The figure shows three views and two pictorial views of one solid part (mm, origin at its lowest corner). Answer the questions. Coordinates: 2 decimals unless noted, no trailing zeros. Order: outer loops, then holes, each group sorted by start corner. A loop starts at its lowest first (then second) coordinate and runs counter-clockwise, first axis right, second up.
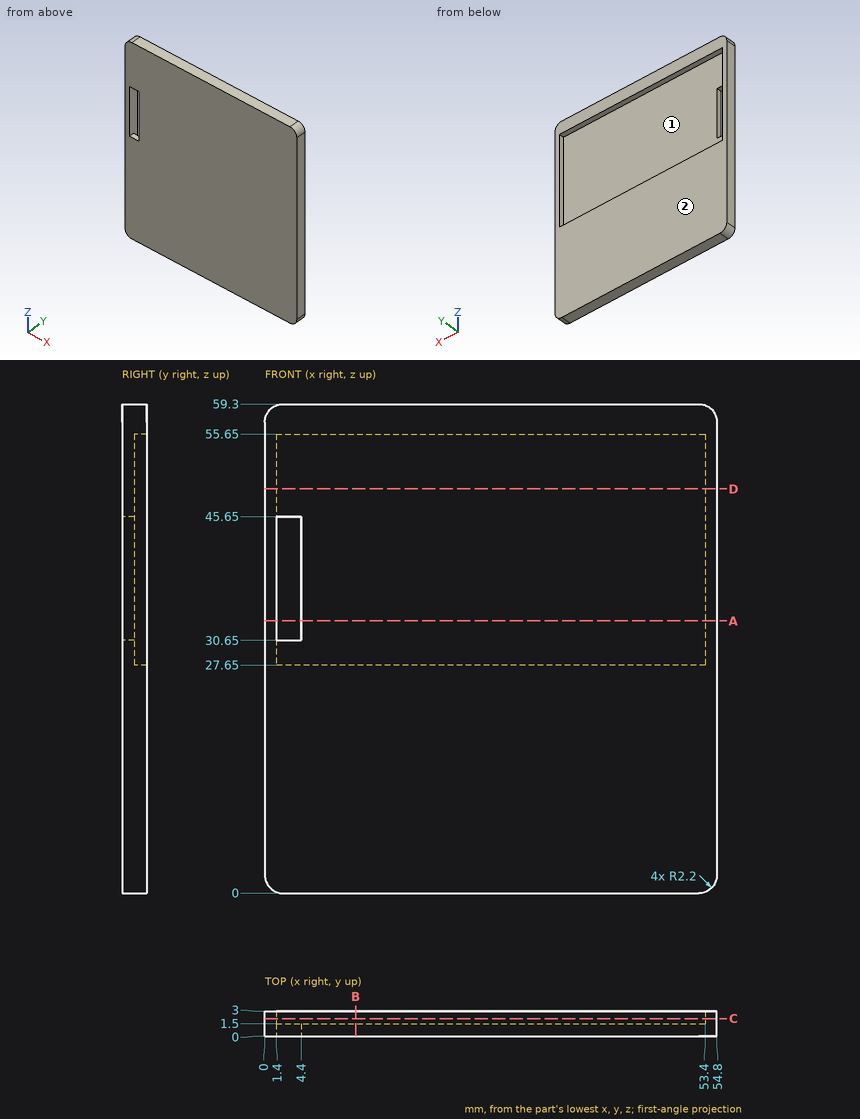
1) A cutting plane is placed at A-A, the plane z = 33. Write down the section's boundary in (x, y), plus the area to 3 significant figures.
2) A cutting plane is placed at D-D, the plane z = 49. Write down the section's boundary in (x, y), plus the area to 3 significant figures.
3) A cutting plane is placed at C-C, the plane y = 2.1. Write down the section's boundary in (x, z), plus the area to 3 significant figures.
4) The mould has two halves that part along Z. Classify the marked faces 1 and 2: released by +Z, released by -Z, zero draft, split by the parting line, or undercut.
5) Straight lines are drawn through the part: probe 1 along Z at (x, y) = (50, 2.4); probe 2 along Z at (x, y) = (3, 1.3); probe 3 along X at (y, z) = (2.45, 46). For each, find the intervals that lie inside material, in ascending order.
6) A cutting plane is placed at B-B, the plane x = 11. Write down the section's boundary in (y, z), plus the area to 3 significant figures.
Working result:
1. outline: (0, 0) - (1.4, 0) - (1.4, 3) - (0, 3) - close; (4.4, 0) - (54.8, 0) - (54.8, 3) - (53.4, 3) - (53.4, 1.5) - (4.4, 1.5) - close
1. area: 81.9 mm2
2. outline: (0, 0) - (54.8, 0) - (54.8, 3) - (53.4, 3) - (53.4, 1.5) - (1.4, 1.5) - (1.4, 3) - (0, 3) - close
2. area: 86.4 mm2
3. outline: (0, 2.2) arc R2.2 ccw to (2.2, 0) - (52.6, 0) arc R2.2 ccw to (54.8, 2.2) - (54.8, 57.1) arc R2.2 ccw to (52.6, 59.3) - (2.2, 59.3) arc R2.2 ccw to (0, 57.1) - close; hole (1.4, 27.65) - (53.4, 27.65) - (53.4, 55.65) - (1.4, 55.65) - close
3. area: 1,790 mm2
4. face 1: undercut
4. face 2: zero draft
5. probe 1: z = 0 to 27.65, 55.65 to 59.3
5. probe 2: z = 0 to 30.65, 45.65 to 59.3
5. probe 3: x = 0 to 1.4, 53.4 to 54.8
6. outline: (0, 0) - (3, 0) - (3, 27.65) - (1.5, 27.65) - (1.5, 55.65) - (3, 55.65) - (3, 59.3) - (0, 59.3) - close
6. area: 136 mm2
